Source: three-view drawing plus pictorial views. Frame: mm from the lowest corner of the part. Coordinates: 2 decimals unless noted, no trailing zeros. Write each loop counter-clockwise with the first axis right and the second up, starting at its lowest first coordinate (ties: lowest second). Pieces come first, ordered by that corner, then holes. Notation, with made-up numbers: M 84.25,-34 L 108.25,-34 A15 cw 108.25,-6 Z; hole C -12,43.5 d2. An arc over 180 degrees is marked long. Answer as a JSON object with one key per item and string values. Group by question number.
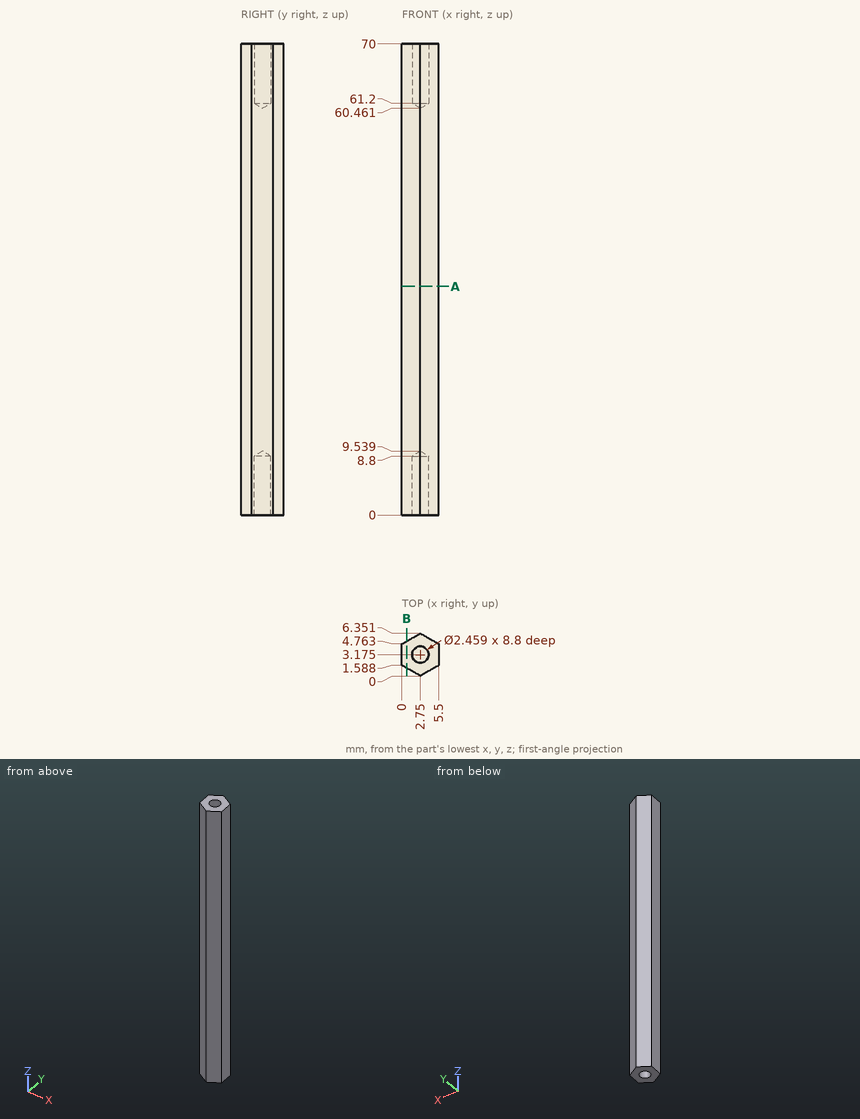
Q1. Pin query (flat end, axial travel): pin 1 Ø3 at (x, y) = (2.75, 3.18) entering from +Z. Return the tip coordinate at first contact, or that it passes through.
Q2. Section A-A, the plane z = 34. Return the cut outline in (x, y), and give its area (3 significant figures).
Q3. Section B-B, the plane x = 0.7. Return the cut outline in (y, z).
Q4. Line query: line 1 (X direction, y = 3, z = 66.5); line 2 (X direction, y = 3.5, z = 61.5) (1 decimal); line 3 (Z direction, x = 1.95, y = 3) (1 decimal). Output: solid intervals per line, ascending. Write a range as from..to.
Filled in:
{
 "1": {"pin 1": "z = 70"},
 "2": {"outline": "M 0,1.59 L 2.75,0 L 5.5,1.59 L 5.5,4.76 L 2.75,6.35 L 0,4.76 Z", "area": "26.2 mm^2"},
 "3": {"outline": "M 1.18,0 L 5.17,0 L 5.17,70 L 1.18,70 Z"},
 "4": {"line 1": "0..1.53, 3.97..5.5", "line 2": "0..1.6, 3.9..5.5", "line 3": "9..61"}
}
